For this review, take the finished solid that the model builds, in its own axes (mm). Face numbers are marked on the shaded views. A direction names the side the tool comes from. Coordinates: 2 decimals unless noted, no trailing zeros. Loops run counter-clockwise (first coordinate to the right, second up) from the corner with the lowest first, then second, coordinate; pieces in that order, holes last.
1. Mouldability with a two-part tool opening along X and no side actions: class the marked faces 1, 2 and 3 as pulls with the +X half, pulls with the -X half, needs draft (parallel to the pull), parting line crosses it, or undercut.
2. Take a section at A-A, the plane z = 9.75. State the section outline as (x, y) points, then the cut area to 3 significant figures.
3. Take a section at D-D, the plane y = 1.5. State the section outline as (x, z) points, then the cut area to 3 significant figures.
4. Machinability: for the marked faces 4, 5 and 6, which of the approach directions +Z, -Z, +X, -X, +Y, -Y give a long, thin tool a straight path to every point of the face, cutting with its end or side? Answer none if there is none.
5. Clearance check with flat-ended pins moving along their axes: P1, Ø9.5, axis at y = 14.5, z = 8.5, coming from the +X side; P2, Ø8, axis at x = 0.5, y = -6, coming from the +Z side; P3, Ø1, axis at x = 18.5, z = 12, coming from the +Y side; P4, Ø9.5, axis at y = 2, z = 5.5, coming from the -X side. State where each tip first meets the part, or that it passes through.
6. Take a section at C-C, the plane x = -23. State the section outline as (y, z) points, then the cut area to 3 significant figures.
7. Take a section at B-B, the plane y = -6. State the section outline as (x, z) points, then the cut area to 3 significant figures.
8. To check wall thickness, follow probe 1 along X at (y, z) = (9, 16); probe 2 along X at (y, z) = (5.5, 8.75); probe 3 along Y at (x, z) = (-11.5, 7.5). State the ranges of each line that lie inside material, in increasing order.
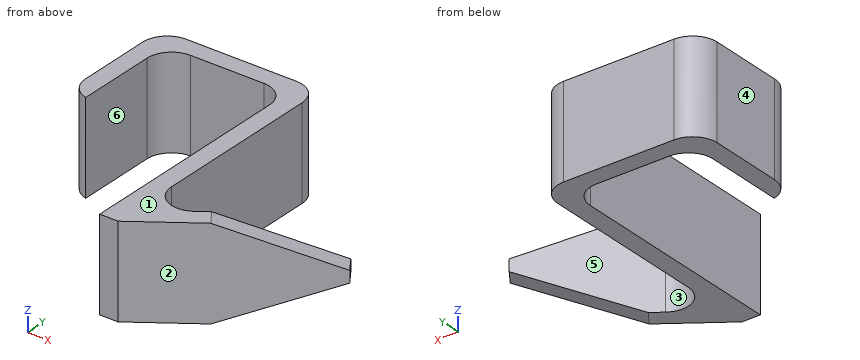
```python
from build123d import *

# Parameters (mm, degrees)
F1_DEPTH     = 19.05
F2_T1_DEPTH  = 19.05
F2_T3_DEPTH  = 19.05
F2_T5_DEPTH  = 19.05
F2_T7_DEPTH  = 44.45
F2_T9_DEPTH  = 44.45
F2_T11_DEPTH = 43.6434442484
F3_SIZE2     = 8.3203595553
F3_SIZE      = 22.86
F3_2_SIZE2   = 8.3203595553
F3_2_SIZE    = 22.86


# Not quite as in the source:
# - a fillet or chamfer that OpenCascade refuses, or shapes differently, is made with other operations: its cross-section is extruded or revolved along the edge and cut away or added


with BuildPart() as f1:
    # F0 (on Top) → F1 (new body)
    with BuildSketch(Plane.XY):
        Polygon((-33.02, 29.6357684863), (-33.02, 4.2357684863), (-29.21, 4.2357684863), (-29.21, 25.8257684863), (-3.81, 25.8257684863), (-3.81, -24.9742315137), (0, -24.9742315137), (31.2096928874, -3.1209692887), (29.0243666649, 0), (0, -20.3230803305), (0, 29.6357684863), align=None)
    extrude(amount=F1_DEPTH)

    # F2: fillet of radius 5.08 on 6 edges, made by hand

    # F2_s2 → F2_t1 (join)
    with BuildSketch(Plane.XY):
        with BuildLine():
            ThreePointArc((7.9937682967, -14.7257835105), (2.7343170448, -15.0705061581), (0, -10.5644911255))
            Line((0, -10.5644911255), (0, -20.3230803305))
            Line((0, -20.3230803305), (7.9937682967, -14.7257835105))
        make_face()
    extrude(amount=F2_T1_DEPTH)

    # F2_s4 → F2_t3 (join)
    with BuildSketch(Plane.XY):
        with BuildLine():
            ThreePointArc((-29.21, 20.7457684863), (-27.7221024484, 24.3378709347), (-24.13, 25.8257684863))
            Line((-24.13, 25.8257684863), (-29.21, 25.8257684863))
            Line((-29.21, 25.8257684863), (-29.21, 20.7457684863))
        make_face()
    extrude(amount=F2_T3_DEPTH)

    # F2_s6 → F2_t5 (join)
    with BuildSketch(Plane.XY):
        with BuildLine():
            ThreePointArc((-8.89, 25.8257684863), (-5.2978975516, 24.3378709347), (-3.81, 20.7457684863))
            Line((-3.81, 20.7457684863), (-3.81, 25.8257684863))
            Line((-3.81, 25.8257684863), (-8.89, 25.8257684863))
        make_face()
    extrude(amount=F2_T5_DEPTH)

    # F2_s8 → F2_t7 (cut)
    with BuildSketch(Plane.XY.offset(-12.7)):
        with BuildLine():
            ThreePointArc((0, 24.5557684863), (-1.4878975516, 28.1478709347), (-5.08, 29.6357684863))
            Line((-5.08, 29.6357684863), (0, 29.6357684863))
            Line((0, 29.6357684863), (0, 24.5557684863))
        make_face()
    extrude(amount=F2_T7_DEPTH, mode=Mode.SUBTRACT)

    # F2_s10 → F2_t9 (cut)
    with BuildSketch(Plane.XY.offset(-12.7)):
        with BuildLine():
            ThreePointArc((-33.02, 24.5557684863), (-31.5321024484, 28.1478709347), (-27.94, 29.6357684863))
            Line((-27.94, 29.6357684863), (-33.02, 29.6357684863))
            Line((-33.02, 29.6357684863), (-33.02, 24.5557684863))
        make_face()
    extrude(amount=F2_T9_DEPTH, mode=Mode.SUBTRACT)

    # F2_s12 → F2_t11 (cut)
    with BuildSketch(Plane.XY.offset(-12.2967221242)):
        with BuildLine():
            ThreePointArc((-29.21, 4.2357684863), (-31.9560926284, 6.0436053626), (-33.02, 9.154457336))
            Line((-33.02, 9.154457336), (-33.02, 4.2357684863))
            Line((-33.02, 4.2357684863), (-29.21, 4.2357684863))
        make_face()
    extrude(amount=F2_T11_DEPTH, mode=Mode.SUBTRACT)

    # F3
    f3_edges = [f1.edges().sort_by_distance(p)[0] for p in [
        (30.11703, -1.560485, 19.05),
    ]]
    f3_side = f1.faces().sort_by_distance((-2.966928, -2.114232, 19.05))[0]
    chamfer(f3_edges, length=F3_SIZE, length2=F3_SIZE2, reference=f3_side)

    # F3#2
    f3_2_edges = [f1.edges().sort_by_distance(p)[0] for p in [
        (30.11703, -1.560485, 0),
    ]]
    f3_2_side = f1.faces().sort_by_distance((-2.966928, -2.114232, 0))[0]
    chamfer(f3_2_edges, length=F3_2_SIZE, length2=F3_2_SIZE2, reference=f3_2_side)


solid = f1.part
```
Results list:
1. face 1: needs draft
1. face 2: pulls with the +X half
1. face 3: undercut
2. outline: (-33.02, 9.15) arc R5.08 ccw to (-29.21, 4.24) - (-29.21, 20.75) arc R5.08 cw to (-24.13, 25.83) - (-8.89, 25.83) arc R5.08 cw to (-3.81, 20.75) - (-3.81, -24.97) - (0, -24.97) - (31.21, -3.12) - (29.02, 0) - (7.99, -14.73) arc R5.08 cw to (0, -10.56) - (0, 24.56) arc R5.08 ccw to (-5.08, 29.64) - (-27.94, 29.64) arc R5.08 ccw to (-33.02, 24.56) - close
2. area: 558 mm2
3. outline: (-3.81, 0) - (0, 0) - (0, 19.05) - (-3.81, 19.05) - close
3. area: 72.6 mm2
4. face 4: +Z, -Z, -X, +Y, -Y
4. face 5: +Z, -Z, +Y
4. face 6: +Z, -Z, -Y
5. P1: stops at x = 0
5. P2: stops at z = 19.05
5. P3: stops at y = -7.02
5. P4: stops at x = -32.41
6. outline: (25.83, 0) - (29.64, 0) - (29.64, 19.05) - (25.83, 19.05) - close
6. area: 72.6 mm2
7. outline: (-3.81, 0) - (0, 0) - (0, 19.05) - (-3.81, 19.05) - close; (20.46, 4.51) - (27.1, 6.49) - (27.1, 12.56) - (20.46, 14.54) - close
7. area: 126 mm2
8. probe 1: x = -33.02 to -29.21, -3.81 to 0
8. probe 2: x = -31.47 to -29.21, -3.81 to 0
8. probe 3: y = 25.83 to 29.64
